Part model, mm, in its own coordinate system. Face numbers are marked on the shaded views. A direction names the side the tool comes from. Round coordinates to 2 decimals unless told otherwise and drop trailing zeros. Loops run counter-clockwise (first coordinate to the right, second up) from the corner with the lowest first, then second, coordinate; pieces in that order, holes last.
1) Probe line 1 (X direction, y = 0, z = -7); line 2 (Z direction, x = -3.5, y = -4.5); line 3 (Y direction, x = -3.5, z = 0.25). List the from-to ranges inside material, lowest first.
2) Drop flat-ended pins along their axis: P1, Ø2, axis at y = 1.5, z = -3.5, coming from the +X side; P2, Ø1, axis at y = 4.5, z = -8.5, coming from the +X side; P3, Ø4, axis at x = -4, z = -3, coming from the -Y side; P4, Ø1.5, axis at x = -3, z = 1.5, coming from the -Y side. Give the stop position or say it passes through.
3) Band-saw the part on C-C, the plane z = -4. Write the cut outline in (x, y), then the cut area to 3 significant figures.
4) 3-axis set-ups, long thin cutter, end or side, ignore diameter. For the marked faces 4, 5, 6 and 7: which of +Z, -Z, +X, -X, +Y, -Y reach the whole face in a straight line?
5) Band-saw the part on B-B, the plane y = 0. Write the cut outline in (x, z), then the cut area to 3 significant figures.
6) Band-saw the part on A-A, the plane x = 0. Write the cut outline in (y, z), then the cut area to 3 significant figures.
7) Band-saw the part on D-D, the plane y = -4.5. Write the cut outline in (x, z), then the cut area to 3 significant figures.
8) Mould opens along Y. For the marked faces 1, 2 and 3 say: +Y half, -Y half, draft (parallel to the pull), parting line (faces both ways), or undercut.
from build123d import *

# Parameters (mm, degrees)
SKETCH_1_R               = 7
EXTRUDE_1_DEPTH          = 4
SKETCH_2_R               = 5.15
EXTRUDE_2_DEPTH          = 11
SKETCH_3_R               = 4
CUT_EXTRUDE_1_DEPTH      = 1
CUT_EXTRUDE_1_DEPTH_BACK = 16
SKETCH_6_W               = 4.3
SKETCH_6_H               = 3.4
CUT_EXTRUDE_2_DEPTH      = 8
CUT_EXTRUDE_2_DEPTH_BACK = 8


with BuildPart() as part:
    # 草图1 → 凸台-拉伸1 (new body)
    with BuildSketch(Plane.XY):
        Circle(SKETCH_1_R)
    extrude(amount=EXTRUDE_1_DEPTH)

    # 草图2 → 凸台-拉伸2 (add)
    with BuildSketch(Plane(origin=(0, 0, 0), x_dir=(-1, 0, 0), z_dir=(0, 0, -1))):
        Circle(SKETCH_2_R)
    extrude(amount=EXTRUDE_2_DEPTH)

    # 草图3 → 切除-拉伸1 (cut, two sides)
    with BuildSketch(Plane(origin=(0, 0, -11), x_dir=(-1, 0, 0), z_dir=(0, 0, -1))) as cut_extrude_1_sk:
        Circle(SKETCH_3_R)
    extrude(amount=CUT_EXTRUDE_1_DEPTH, mode=Mode.SUBTRACT)
    extrude(cut_extrude_1_sk.sketch, amount=-CUT_EXTRUDE_1_DEPTH_BACK, mode=Mode.SUBTRACT)

    # 草图6 → 切除-拉伸2 (cut, two sides)
    with BuildSketch(Plane(origin=(0, 0, 0), x_dir=(0, 0, -1), z_dir=(1, 0, 0))) as cut_extrude_2_sk:
        with Locations((8.85, 3.45)):
            Rectangle(SKETCH_6_W, SKETCH_6_H)
        with Locations((8.85, -3.45)):
            Rectangle(SKETCH_6_W, SKETCH_6_H)
    extrude(amount=CUT_EXTRUDE_2_DEPTH, mode=Mode.SUBTRACT)
    extrude(cut_extrude_2_sk.sketch, amount=-CUT_EXTRUDE_2_DEPTH_BACK, mode=Mode.SUBTRACT)


solid = part.part
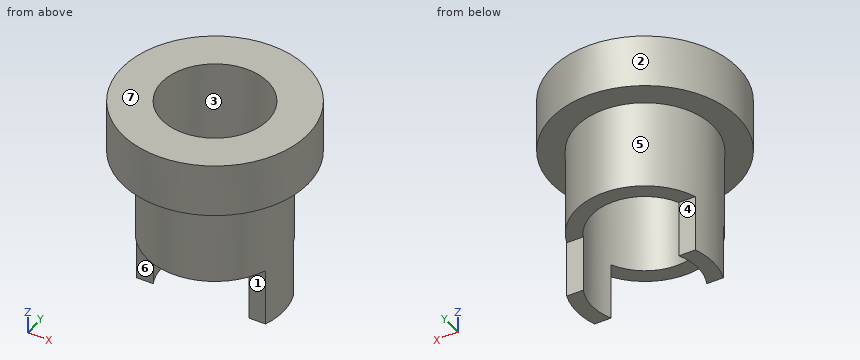
Reported:
1. line 1: x = -5.15 to -4, 4 to 5.15
1. line 2: z = 0 to 4
1. line 3: y = -6.06 to -1.94, 1.94 to 6.06
2. P1: stops at x = 5.13
2. P2: passes through
2. P3: stops at y = -4.75
2. P4: stops at y = -6.63
3. outline: circle Ø10.3 at (0, 0); hole circle Ø8 at (0, 0)
3. area: 33.1 mm2
4. face 4: -Z, +X, -X, +Y
4. face 5: -Z
4. face 6: -Z, +X, -X, -Y
4. face 7: +Z, +X, -X, +Y, -Y
5. outline: (-7, 0) - (-5.15, 0) - (-5.15, -11) - (-4, -11) - (-4, 4) - (-7, 4) - close; (4, -11) - (5.15, -11) - (5.15, 0) - (7, 0) - (7, 4) - (4, 4) - close
5. area: 49.3 mm2
6. outline: (-7, 0) - (-5.15, 0) - (-5.15, -6.7) - (-4, -6.7) - (-4, 4) - (-7, 4) - close; (4, -6.7) - (5.15, -6.7) - (5.15, 0) - (7, 0) - (7, 4) - (4, 4) - close
6. area: 39.4 mm2
7. outline: (-5.36, 0) - (-2.5, 0) - (-2.5, -6.7) - (2.5, -6.7) - (2.5, 0) - (5.36, 0) - (5.36, 4) - (-5.36, 4) - close
7. area: 76.5 mm2
8. face 1: -Y half
8. face 2: parting line
8. face 3: undercut
